```python
from build123d import *

# Parameters (mm, degrees)
SKETCH1_W               = 279.4
SKETCH1_H               = 76.2
BOSS_EXTRUDE1_DEPTH     = 3
SKETCH3_W               = 3
SKETCH3_H               = 7.8
CUT_EXTRUDE1_DEPTH      = 145.833352512
LPATTERN1_COUNT         = 4
LPATTERN1_PITCH         = 22.8
MIRROR1_COPY_1_SKETCH_W = 3
MIRROR1_COPY_1_SKETCH_H = 7.8
MIRROR1_COPY_1_DEPTH    = 145.833352512
MIRROR1_COPY_2_SKETCH_W = 3
MIRROR1_COPY_2_SKETCH_H = 7.8
MIRROR1_COPY_2_DEPTH    = 145.833352512
MIRROR1_COPY_3_SKETCH_W = 3
MIRROR1_COPY_3_SKETCH_H = 7.8
MIRROR1_COPY_3_DEPTH    = 145.833352512
SKETCH4_W               = 3
SKETCH4_H               = 15
CUT_EXTRUDE2_DEPTH      = 10
LPATTERN2_COUNT         = 3
LPATTERN2_PITCH         = 22.8
MIRROR2_COPY_1_SKETCH_W = 3
MIRROR2_COPY_1_SKETCH_H = 15
MIRROR2_COPY_1_DEPTH    = 10
MIRROR2_COPY_2_SKETCH_W = 3
MIRROR2_COPY_2_SKETCH_H = 15
MIRROR2_COPY_2_DEPTH    = 10
SKETCH5_W               = 3
SKETCH5_H               = 7.8
BOSS_EXTRUDE2_DEPTH     = 3
LPATTERN3_COUNT         = 8
LPATTERN3_PITCH         = 22.8


with BuildPart() as part:
    # Sketch1 → Boss-Extrude1 (new body)
    with BuildSketch(Plane(origin=(0, 0, 0), x_dir=(0, 0, -1), z_dir=(1, 0, 0))):
        Rectangle(SKETCH1_W, SKETCH1_H)
    extrude(amount=-BOSS_EXTRUDE1_DEPTH)

    # Sketch3 → Cut-Extrude1 (cut, through all)
    with BuildSketch(Plane.ZY.offset(3)):
        with Locations((-138.2, 34.2)):
            Rectangle(SKETCH3_W, SKETCH3_H)
    cut_extrude1 = extrude(amount=-CUT_EXTRUDE1_DEPTH, mode=Mode.SUBTRACT)

    # LPattern1: Cut-Extrude1 ×4
    with Locations(*[(0, -i * LPATTERN1_PITCH, 0) for i in range(1, LPATTERN1_COUNT)]):
        add(cut_extrude1, mode=Mode.SUBTRACT)

    # Mirror1: Cut-Extrude1 across plane
    add(cut_extrude1.mirror(Plane.XY), mode=Mode.SUBTRACT)

    # Mirror1 copy 1 sketch → Mirror1 copy 1 (cut, through all)
    with BuildSketch(Plane(origin=(-3, -22.8, 0), x_dir=(0, 0, -1), z_dir=(-1, 0, 0))):
        with Locations((-138.2, -34.2)):
            Rectangle(MIRROR1_COPY_1_SKETCH_W, MIRROR1_COPY_1_SKETCH_H)
    extrude(amount=-MIRROR1_COPY_1_DEPTH, mode=Mode.SUBTRACT)

    # Mirror1 copy 2 sketch → Mirror1 copy 2 (cut, through all)
    with BuildSketch(Plane(origin=(-3, -45.6, 0), x_dir=(0, 0, -1), z_dir=(-1, 0, 0))):
        with Locations((-138.2, -34.2)):
            Rectangle(MIRROR1_COPY_2_SKETCH_W, MIRROR1_COPY_2_SKETCH_H)
    extrude(amount=-MIRROR1_COPY_2_DEPTH, mode=Mode.SUBTRACT)

    # Mirror1 copy 3 sketch → Mirror1 copy 3 (cut, through all)
    with BuildSketch(Plane(origin=(-3, -68.4, 0), x_dir=(0, 0, -1), z_dir=(-1, 0, 0))):
        with Locations((-138.2, -34.2)):
            Rectangle(MIRROR1_COPY_3_SKETCH_W, MIRROR1_COPY_3_SKETCH_H)
    extrude(amount=-MIRROR1_COPY_3_DEPTH, mode=Mode.SUBTRACT)

    # Sketch4 → Cut-Extrude2 (cut)
    with BuildSketch(Plane(origin=(0, 0, 0), x_dir=(0, 0, -1), z_dir=(1, 0, 0))):
        with Locations((-95.2, 22.8)):
            Rectangle(SKETCH4_W, SKETCH4_H)
    cut_extrude2 = extrude(amount=-CUT_EXTRUDE2_DEPTH, mode=Mode.SUBTRACT)

    # LPattern2: Cut-Extrude2 ×3
    with Locations(*[(0, -i * LPATTERN2_PITCH, 0) for i in range(1, LPATTERN2_COUNT)]):
        add(cut_extrude2, mode=Mode.SUBTRACT)

    # Mirror2: Cut-Extrude2 across plane
    add(cut_extrude2.mirror(Plane.XY), mode=Mode.SUBTRACT)

    # Mirror2 copy 1 sketch → Mirror2 copy 1 (cut)
    with BuildSketch(Plane(origin=(0, -22.8, 0), x_dir=(0, 0, 1), z_dir=(1, 0, 0))):
        with Locations((-95.2, -22.8)):
            Rectangle(MIRROR2_COPY_1_SKETCH_W, MIRROR2_COPY_1_SKETCH_H)
    extrude(amount=-MIRROR2_COPY_1_DEPTH, mode=Mode.SUBTRACT)

    # Mirror2 copy 2 sketch → Mirror2 copy 2 (cut)
    with BuildSketch(Plane(origin=(0, -45.6, 0), x_dir=(0, 0, 1), z_dir=(1, 0, 0))):
        with Locations((-95.2, -22.8)):
            Rectangle(MIRROR2_COPY_2_SKETCH_W, MIRROR2_COPY_2_SKETCH_H)
    extrude(amount=-MIRROR2_COPY_2_DEPTH, mode=Mode.SUBTRACT)

    # Sketch5 → Boss-Extrude2 (add)
    with BuildSketch(Plane(origin=(0, 38.1, 0), x_dir=(1, 0, 0), z_dir=(0, 1, 0))):
        with Locations((-1.5, -79.8)):
            Rectangle(SKETCH5_W, SKETCH5_H)
    boss_extrude2 = extrude(amount=BOSS_EXTRUDE2_DEPTH)

    # LPattern3: Boss-Extrude2 ×8
    with Locations(*[(0, 0, -i * LPATTERN3_PITCH) for i in range(1, LPATTERN3_COUNT)]):
        add(boss_extrude2)


solid = part.part
```
The listing builds one solid part. Answer for the finished solid, in the listing's coordinates (mm). Give positions to 0.01 mm unless a question says otherwise; leave off trailing zeros. Order: outer loops, then holes, each group sorted by start corner. A loop starts at its lowest first (then second) coordinate and runs counter-clockwise, first axis right, second up. Notation, with made-up numbers: (76.25, 67.5) - (102.25, 67.5) arc R17 ccw to (102.25, 76.5) - close; hole circle Ø9 at (74, 6.25). An arc over 180 degrees is marked (long way). Answer in a Markdown table with one row per item. Add a question column.
Q1. Given P1, Ø0.9, axis at x = -1.5, y = 39.5, coming from the +Z side; P2, Ø0.9, axis at x = -2, z = 95.5, coming from the +Y side; P3, Ø0.9, axis at x = -1.5, y = -10, coming from the +Z side; P4, Ø4, axis at y = 6.5, z = 7, coming from the +X side, each flat-ended and moving along its own axis, determine where each tip first touches the part or whether it passes through.
Q2. The part is cut by section B-B (x = -0.5). Give the number of separate pieces and of enclosed holes in the cut face, then the cut area to 3 significant figures.
Q3. The part is cut by section A-A (y = -20). Determine the outline of the cut face in (x, z), then the cut area to 3 significant figures.
Q4. Find the intervals of material crossed by line 1 along Z through (x, y) = (-0.9, -19); line 2 along Z through (x, y) = (-2.15, -13); line 3 along Y through (x, z) = (-2.75, -46.5), in increasing order. Write a range as [from, to].
Q5. The part is cut by section C-C (z = 118). Determine the outline of the cut face in (x, y).
Determined:
| question | item | result |
|---|---|---|
| 1 | P1 | stops at z = 83.7 |
| 1 | P2 | stops at y = 38.1 |
| 1 | P3 | stops at z = 136.7 |
| 1 | P4 | stops at x = 0 |
| 2 | separate pieces | 1 |
| 2 | enclosed holes | 6 |
| 2 | area | 21,000 mm² |
| 3 | outline | (-3, -139.7) - (0, -139.7) - (0, -96.7) - (-3, -96.7) - close; (-3, -93.7) - (0, -93.7) - (0, 93.7) - (-3, 93.7) - close; (-3, 96.7) - (0, 96.7) - (0, 139.7) - (-3, 139.7) - close |
| 3 | area | 820 mm² |
| 4 | line 1 | z = [-139.7, -96.7], [-93.7, 93.7], [96.7, 139.7] |
| 4 | line 2 | z = [-136.7, 136.7] |
| 4 | line 3 | y = [-38.1, 38.1] |
| 5 | outline | (-3, -38.1) - (0, -38.1) - (0, 38.1) - (-3, 38.1) - close |
